Here's how the part is built. I have some questions about the finished solid (model axes, mm). Round coordinates to 2 decimals unless told otherwise and drop trailing zeros. Loops run counter-clockwise (first coordinate to the right, second up) from the corner with the lowest first, then second, coordinate; pieces in that order, holes last. Notation, with made-up numbers: M 87,3.5 L 92,3.5 A15 ccw 92,23.5 Z; hole C 8,85 d3. An arc over 180 degrees is marked long. Write each question's results on one line, items separated by ' | '. Start each with the question number.
```python
from build123d import *

# Parameters (mm, degrees)
EXTRUDE_1_DEPTH     = 4
SKETCH_2_R          = 3
CUT_EXTRUDE_1_DEPTH = 10


with BuildPart() as part:
    # 草图1 → 凸台-拉伸1 (new body)
    with BuildSketch(Plane.XY):
        Polygon((-85, -75), (100, -75), (100, -2.031815791), (60, -2.031815791), (60, 17.968184209), (25, 57.968184209), (25, 147), (-35, 147), (-85, 97), align=None)
    extrude(amount=EXTRUDE_1_DEPTH)

    # 草图2 → 切除-拉伸1 (cut)
    with BuildSketch(Plane(origin=(0, 0, 0), x_dir=(-1, 0, 0), z_dir=(0, 0, -1))):
        with Locations((75, -65)):
            Circle(SKETCH_2_R)
        with Locations((-50, 7.332157467)):
            Circle(SKETCH_2_R)
        with Locations((9.393398282, 137)):
            Circle(SKETCH_2_R)
        with Locations((75, 60.786796564)):
            Circle(SKETCH_2_R)
    extrude(amount=-CUT_EXTRUDE_1_DEPTH, mode=Mode.SUBTRACT)


solid = part.part
```
Item 1: If we section it at D-D on z = 1.3: Please give me the cut outline in (x, y).
Item 2: I'm going to push flat-ended pins straight in: pin 1 (1 mm diameter, centred on x = -11, y = 31, fed in from -Z); pin 2 (2 mm diameter, centred on y = 6.5, z = 3, fed in from +X); pin 3 (3.5 mm diameter, centred on x = 50, y = 7.33, fed in from +Z). Where does each tip first touch, or does it pass through?
Item 3: If we section it at A-A on y = -65: Please give me the cut outline in (x, z).
Item 4: If we section it at C-C on x = 50: Please give me the cut outline in (y, z).
Item 5: If we mould it in two halves opening along Y, with no side actions, what happens to faces 1 (the face through (-11.006, 139.53, 1.972)), 2 (the face through (-14, 13, 0)), 3 (the face through (-72.6, -66.8, 2)), 4 (the face through (-60, 122, 2))? For each: released by +Y, released by -Y, zero draft, split by the parting line, or undercut.
Item 6: If we section it at B-B on x = -75: Please give me the cut outline in (y, z).
Item 7: I need wall thicknesses on L1, parallel to Y at x = -75, z = 1.85; L2, parallel to Y at x = 66.5, z = 0.4; L3, parallel to X at y = 84, z = 0.45. Which ranges of each line are inside material? Lowest first, please.
Numbers:
1) outline: M -85,-75 L 100,-75 L 100,-2.03 L 60,-2.03 L 60,17.97 L 25,57.97 L 25,147 L -35,147 L -85,97 Z; hole C -75,-65 d6; hole C -75,60.79 d6; hole C -9.39,137 d6; hole C 50,7.33 d6
2) pin 1: z = 0 | pin 2: x = 60 | pin 3: through
3) outline: M -85,0 L -78,0 L -78,4 L -85,4 Z; M -72,0 L 100,0 L 100,4 L -72,4 Z
4) outline: M -75,0 L 4.33,0 L 4.33,4 L -75,4 Z; M 10.33,0 L 29.4,0 L 29.4,4 L 10.33,4 Z
5) face 1: undercut | face 2: zero draft | face 3: undercut | face 4: released by +Y
6) outline: M -75,0 L -68,0 L -68,4 L -75,4 Z; M -62,0 L 57.79,0 L 57.79,4 L -62,4 Z; M 63.79,0 L 107,0 L 107,4 L 63.79,4 Z
7) L1: -75 to -68, -62 to 57.79, 63.79 to 107 | L2: -75 to -2.03 | L3: -85 to 25
